from build123d import *

# Parameters (mm, degrees)
F0_R     = 29.5
F2_DEPTH = 10
F3_D     = 57
F5_R     = 29.5
F6_DEPTH = 3


with BuildPart() as f2:
    # F0 (on Top) → F2 (new body)
    with BuildSketch(Plane.XY):
        Circle(F0_R)
    extrude(amount=F2_DEPTH)

    # F3 (through all)
    with Locations(Plane(origin=(0, 0, 0), x_dir=(1, 0, 0), z_dir=(0, 0, -1))):
        with Locations((0, 0)):
            Hole(F3_D / 2)

    # F5 (on offset) → F6 (join)
    with BuildSketch(Plane.XY.offset(-3)):
        Circle(F5_R)
    extrude(amount=F6_DEPTH)


solid = f2.part
CAD build for the part. Positions are in the model's coordinates, mm. A direction names the side the tool comes from. Coordinates: 2 decimals unless noted, no trailing zeros. Loops run counter-clockwise (first coordinate to the right, second up) from the corner with the lowest first, then second, coordinate; pieces in that order, holes last. Notation, with made-up numbers: (-4, 86.25) - (46, 86.25) arc R18 ccw to (46, 109.25) - close; hole circle Ø11 at (-32, -15). An arc over 180 degrees is marked (long way). Use one line per item in the form item = value. Start each with the question number.
1) Flat gauge pins, fed straight in: pin 1 (1.5 mm diameter, centred on y = 11, z = 0.5, fed in from -X); pin 2 (5 mm diameter, centred on y = -10, z = 7, fed in from -X); pin 3 (2 mm diameter, centred on x = -9, z = 2, fed in from -Y). Where does each tip first touch, or does it go through?
2) Band-saw the part on C-C (z = 2.75). Give the cut face in (x, y), and give its area (3 significant figures).
3) Band-saw the part on A-A (x = 0). Give the cut face in (y, z), and give its area (3 significant figures).
4) Two-plate mould, pull along Y, no slides. Class faces 3 (the face through (-26.327, 10.916, 5.07)), 4 (the face through (-15.4, 24.2, 10)), 5 (the face through (28.14, 8.86, 3.41)): +Y half, -Y half, draft (parallel to the pull), parting line (faces both ways), or undercut.
5) Tool access for faces 1 (the face through (0, 0, 0)), 2 (the face through (0, 0, -3)): list every direction of +Z, -Z, +X, -X, +Y, -Y with a clear straight run to the whole face (end or side of a thin tool).
6) Drill centre lines: L1, parallel to Y at x = 0, z = 7.5; L2, parallel to Z at x = 4, y = 26; L3, parallel to Y at x = 11, z = 6. Where is each one in solid material? Low to high. Write a range as from..to.
Check values:
q1.pin_1 = -27.66
q1.pin_2 = -28.53
q1.pin_3 = -28.39
q2.outline = circle Ø59 at (0, 0); hole circle Ø57 at (0, 0)
q2.area = 182 mm2
q3.outline = (-29.5, -3) - (29.5, -3) - (29.5, 10) - (28.5, 10) - (28.5, 0) - (-28.5, 0) - (-28.5, 10) - (-29.5, 10) - close
q3.area = 197 mm2
q4.face_3 = undercut
q4.face_4 = draft
q4.face_5 = parting line
q5.face_1 = +Z
q5.face_2 = -Z, +X, -X, +Y, -Y
q6.L1 = -29.5..-28.5, 28.5..29.5
q6.L2 = -3..0
q6.L3 = -27.37..-26.29, 26.29..27.37
